Autodesk Inventor part; units mm, degrees
ref_plane "YZ Plane" through (0, 0, 0) normal (1, 0, 0) x (0, 1, 0)
ref_plane "XZ Plane" through (0, 0, 0) normal (0, 1, 0) x (-1, 0, 0)
ref_plane "XY Plane" through (0, 0, 0) normal (0, 0, 1) x (1, 0, 0)
sketch "Boceto1" plane through (0, 0, 0) normal (0, 0, 1) x (1, 0, 0)
  circle A0 centre (0, 0) radius 3
  circle A1 centre (0, 0) radius 5
  dimension "d0" = 6
  dimension "d1" = 10
extrude "Extrusión1" add sketch "Boceto1" along normal blind 30 contours A0
extrude "Extrusión2" add sketch "Boceto1" against normal blind 6 contours A0 | A1
thread "Rosca1"
sketch "Boceto2" plane through (0, 0, -6) normal (0, 0, -1) x (-1, 0, 0)
  line L0 (3, 0) -> (1.5, -2.5981)
  line L1 (1.5, -2.5981) -> (-1.5, -2.5981)
  line L2 (-1.5, -2.5981) -> (-3, 0)
  line L3 (-3, 0) -> (-1.5, 2.5981)
  line L4 (-1.5, 2.5981) -> (1.5, 2.5981)
  line L5 (1.5, 2.5981) -> (3, 0)
  point P0 (0, 0)
  point P1 (0, 0)
  dimension "d8" = 6
extrude "Extrusión3" cut sketch "Boceto2" against normal blind 4
properties part number "tornilloM6x30mm" material "Hierro, dúctil"
Verification items for the finished model (mm, model axes). A direction names the side the tool comes from. Give positions to 0.01 mm unless a question says otherwise; leave off trailing zeros. Write each loop counter-clockwise with the first axis right and the second up, starting at its lowest first coordinate (ties: lowest second). Pieces come first, ordered by that corner, then holes.
(1) Gauge pin test, flat ends, axial feed: pin 1 (2 mm diameter, centred on y = 1, z = 6.5, fed in from -X); pin 2 (1.5 mm diameter, centred on y = 2, z = 0, fed in from +X); pin 3 (6 mm diameter, centred on x = 0.5, z = 6, fed in from +Y). Record the tip position at first contact, or that the pin passes through.
(2) Mould release check, pull along X, two halves, no side actions. Record for faces 4 (the face through (-2.26, -1.28, -4.03)), 5 (the face through (2.2, -2.2, -6)), 6 (the face through (0, 0, -2)), 7 (the face through (-3, 0, 15)): +X half, -X half, draft (parallel to the pull), parting line (faces both ways), or undercut.
(3) Cross-section at A-A (x = 0). Enter the section's corners in (y, z).
(4) Cross-section at C-C (y = -1.5). Enter the section's corners in (x, z), plus the area to 3 significant figures.
(5) Cross-section at D-D (x = 4.25). Enter the section's corners in (y, z), plus the area to 3 significant figures.
(6) Access from +Z, -Z, +X, -X, +Y, -Y to the whole of each face (thin tool, end or side, straight path). Record for faces 1 (the face through (3.3, 0.1, 0)), 2 (the face through (0, 0, 30)), 3 (the face through (0, -2.598, -4)).
(7) Cross-section at B-B (z = 1). Enter the section's corners in (x, y).
(8) Material ranges on line 1 (Z direction, x = 2.5, y = -2.5); line 2 (Z direction, x = -2, y = -0.75); line 3 (X direction, y = 1.5, z = 4.5), recorded low to high.
Worked out:
1. pin 1: stops at x = -3
1. pin 2: stops at x = 4.84
1. pin 3: stops at y = 3
2. face 4: undercut
2. face 5: draft
2. face 6: undercut
2. face 7: parting line
3. outline: (-5, -6) - (-2.6, -6) - (-2.6, -2) - (2.6, -2) - (2.6, -6) - (5, -6) - (5, 0) - (3, 0) - (3, 30) - (-3, 30) - (-3, 0) - (-5, 0) - close
4. outline: (-4.77, -6) - (-2.13, -6) - (-2.13, -2) - (2.13, -2) - (2.13, -6) - (4.77, -6) - (4.77, 0) - (2.6, 0) - (2.6, 30) - (-2.6, 30) - (-2.6, 0) - (-4.77, 0) - close
4. area: 196 mm2
5. outline: (-2.63, -6) - (2.63, -6) - (2.63, 0) - (-2.63, 0) - close
5. area: 31.6 mm2
6. face 1: +Z
6. face 2: +Z, +X, -X, +Y, -Y
6. face 3: -Z
7. outline: circle Ø6 at (0, 0)
8. line 1: z = -6 to 0
8. line 2: z = -2 to 30
8. line 3: x = -2.6 to 2.6
